For this review, take the finished solid that the model builds, in its own axes (mm). Round coordinates to 2 decimals unless told otherwise and drop trailing zeros. Write each loop counter-clockwise with the first axis right and the second up, starting at its lowest first coordinate (ties: lowest second). Pieces come first, ordered by that corner, then holes. Notation, with made-up numbers: (67, 18) -> (82, 18) arc R10 cw to (82, 37) -> close; hole circle Ø9 at (68.5, 49). An arc over 180 degrees is marked (long way). Answer as CSV lines item,"result". Start each with the question number.
Item 1: Take a section at C-C on z = -194.5. Give the boundary of the cut face in (x, y), then the cut area to 3 significant figures.
Item 2: For pin 1 Ø0.6 at (x, z) = (1, 260) entering from +Y; pin 2 Ø0.6 at (x, z) = (1, -182.5) entering from +Y; pin 3 Ø1 at (x, y) = (1, 8.5) entering from +Z, all flat-tipped, find the tip position at first contact; note any pin that passes through.
Item 3: Take a section at A-A on y = -65. Give the boundary of the cut face in (x, z), then the cut area to 3 significant figures.
Item 4: Take a section at B-B on z = 60. Give the boundary of the cut face in (x, y).
Item 5: Wall thickness on probe 1 along Z at (x, y) = (0.5, -17); probe 2 along Z at (x, y) = (1.6, -52); probe 3 along Z at (x, y) = (0.3, 22.5): over which ranges is each line inside the solid? List them lowest first. Write a range as from..to.
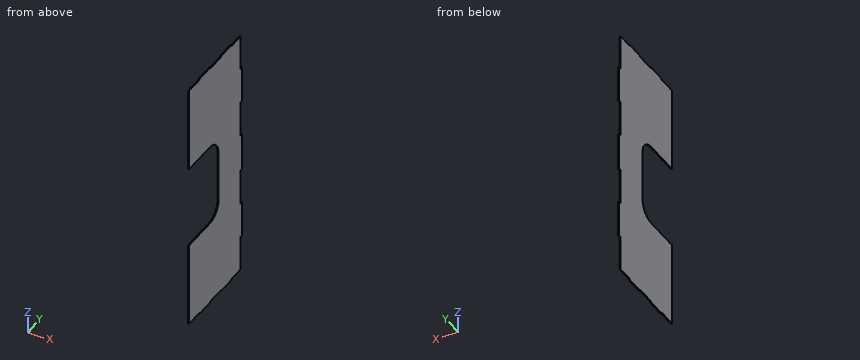
Autodesk Inventor part; units mm, degrees
ref_plane "YZ Plane" through (0, 0, 0) normal (1, 0, 0) x (0, 1, 0)
ref_plane "XZ Plane" through (0, 0, 0) normal (0, 1, 0) x (-1, 0, 0)
ref_plane "XY Plane" through (0, 0, 0) normal (0, 0, 1) x (1, 0, 0)
sketch "Sketch1" plane through (0, 0, 0) normal (1, 0, 0) x (0, 1, 0)
  line L0 (98.4407, 261.352) -> (-81.5593, 261.352)
  line L1 (-81.5593, -230.648) -> (98.4407, -230.648)
  line L2 (98.4407, -230.648) -> (98.4407, 261.352)
  line L3 (-81.5593, 95.352) -> (-11.5593, 95.352)
  line L4 (18.4407, 65.352) -> (18.4407, -34.648)
  line L5 (-11.5593, -64.648) -> (-81.5593, -64.648)
  line L6 (-81.5593, 261.352) -> (-81.5593, 95.352)
  line L7 (-81.5593, -64.648) -> (-81.5593, -230.648)
  arc A0 (18.4407, 65.352) -> (-11.5593, 95.352) centre (-11.5593, 65.352) ccw
  arc A1 (-11.5593, -64.648) -> (18.4407, -34.648) centre (-11.5593, -34.648) ccw
  point P0 (0, 0)
  point P1 (18.4407, -64.648)
  point P2 (18.4407, 95.352)
  dimension "d0" = 180
  dimension "d1" = 492
  dimension "d2" = 100
  dimension "d3" = 160
  dimension "d4" = 166
  dimension "d5" = 100
  dimension "d8" = 30
extrude "Extrusion1" add sketch "Sketch1" along normal blind 2
sketch "Sketch2" plane through (2, 0, 0) normal (1, 0, 0) x (0, 0, -1)
  line L0 (-261.352, 98.4407) -> (-191.352, 98.4407)
  line L1 (-191.352, 98.4407) -> (-191.352, 93.4407)
  line L2 (-191.352, 93.4407) -> (-261.352, 93.4407)
  line L3 (-261.352, 93.4407) -> (-261.352, 98.4407)
  line L4 (230.648, 98.4407) -> (-261.352, 98.4407)
  line L5 (-121.352, 98.4407) -> (-51.352, 98.4407)
  line L6 (-51.352, 98.4407) -> (-51.352, 93.4407)
  line L7 (-51.352, 93.4407) -> (-121.352, 93.4407)
  line L8 (-121.352, 93.4407) -> (-121.352, 98.4407)
  line L9 (20.648, 98.4407) -> (90.648, 98.4407)
  line L10 (90.648, 98.4407) -> (90.648, 93.4407)
  line L11 (90.648, 93.4407) -> (20.648, 93.4407)
  line L12 (20.648, 93.4407) -> (20.648, 98.4407)
  line L13 (160.648, 98.4407) -> (230.648, 98.4407)
  line L14 (230.648, 98.4407) -> (230.648, 93.4407)
  line L15 (230.648, 93.4407) -> (160.648, 93.4407)
  line L16 (160.648, 93.4407) -> (160.648, 98.4407)
  line L17 (230.648, -81.5593) -> (230.648, 98.4407)
  point P0 (0, 0)
  point P1 (230.648, 95.9407)
  point P2 (90.648, 95.9407)
  dimension "d9" = 70
  dimension "d10" = 70
  dimension "d11" = 70
  dimension "d12" = 70
  dimension "d13" = 0
  dimension "d14" = 70
  dimension "d15" = 70
  dimension "d16" = 72
  dimension "d17" = 5
extrude "Extrusion2" cut sketch "Sketch2" against normal blind 2
sketch "Sketch3" plane through (2, 0, 0) normal (1, 0, 0) x (0, 0, -1)
  line L0 (-261.352, 93.4407) -> (-261.352, -81.5593)
  line L1 (-261.352, 93.4407) -> (-259.352, 93.4407)
  line L2 (-259.352, 93.4407) -> (-259.352, 62.4407)
  line L3 (-259.352, 62.4407) -> (-261.352, 62.4407)
  line L4 (-261.352, 62.4407) -> (-261.352, 93.4407)
  line L5 (-261.352, 26.4407) -> (-259.352, 26.4407)
  line L6 (-259.352, 26.4407) -> (-259.352, -9.5593)
  line L7 (-259.352, -9.5593) -> (-261.352, -9.5593)
  line L8 (-261.352, -9.5593) -> (-261.352, 26.4407)
  line L9 (-261.352, -81.5593) -> (-259.352, -81.5593)
  line L10 (-259.352, -81.5593) -> (-259.352, -45.5593)
  line L11 (-259.352, -45.5593) -> (-261.352, -45.5593)
  line L12 (-261.352, -45.5593) -> (-261.352, -81.5593)
  line L13 (64.648, -81.5593) -> (230.648, -81.5593)
  line L14 (230.648, -81.5593) -> (228.648, -81.5593)
  line L15 (228.648, -81.5593) -> (228.648, -45.5593)
  line L16 (228.648, -45.5593) -> (230.648, -45.5593)
  line L17 (230.648, -45.5593) -> (230.648, -81.5593)
  line L18 (230.648, -81.5593) -> (230.648, 93.4407)
  line L19 (230.648, -9.5593) -> (228.648, -9.5593)
  line L20 (228.648, -9.5593) -> (228.648, 26.4407)
  line L21 (228.648, 26.4407) -> (230.648, 26.4407)
  line L22 (230.648, 26.4407) -> (230.648, -9.5593)
  line L23 (160.648, 93.4407) -> (230.648, 93.4407)
  line L24 (230.648, 62.4407) -> (228.648, 62.4407)
  line L25 (228.648, 62.4407) -> (228.648, 93.4407)
  line L26 (228.648, 93.4407) -> (230.648, 93.4407)
  line L27 (230.648, 93.4407) -> (230.648, 62.4407)
  point P0 (0, 0)
  point P1 (-260.352, -9.5593)
  point P2 (-260.352, -45.5593)
  point P3 (-260.352, 62.4407)
  point P4 (-260.352, 26.4407)
  point P5 (229.648, 26.4407)
  point P6 (229.648, 62.4407)
  point P7 (229.648, -9.5593)
  point P8 (229.648, -45.5593)
  dimension "d20" = 36
  dimension "d21" = 36
  dimension "d22" = 36
  dimension "d23" = 36
  dimension "d24" = 2
  dimension "d25" = 2
  dimension "d26" = 36
  dimension "d27" = 36
  dimension "d28" = 36
  dimension "d29" = 36
extrude "Extrusion3" cut sketch "Sketch3" against normal blind 2
properties part number "outer_side"
Output values:
1,outline,"(0, -81.56) -> (2, -81.56) -> (2, 93.44) -> (0, 93.44) -> close"
1,area,"350 mm^2"
2,pin 1,"stops at y = 62.44"
2,pin 2,"stops at y = 93.44"
2,pin 3,"stops at z = 259.35"
3,outline,"(0, -228.65) -> (2, -228.65) -> (2, -64.65) -> (0, -64.65) -> close; (0, 95.35) -> (2, 95.35) -> (2, 259.35) -> (0, 259.35) -> close"
3,area,"656 mm^2"
4,outline,"(0, 18.44) -> (2, 18.44) -> (2, 93.44) -> (0, 93.44) -> close"
5,probe 1,"z = -230.65..-64.65, 95.35..261.35"
5,probe 2,"z = -228.65..-64.65, 95.35..259.35"
5,probe 3,"z = -228.65..259.35"
